Source: three-view drawing plus pictorial views. Frame: mm from the lowest corner of the part. A direction names the side the tool comes from. Give positions to 0.01 mm unless a question says otherwise; leave off trailing zeros. Loops run counter-clockwise (first coordinate to the right, second up) from the corner with the lowest first, then second, coordinate; pieces in that order, holes last.
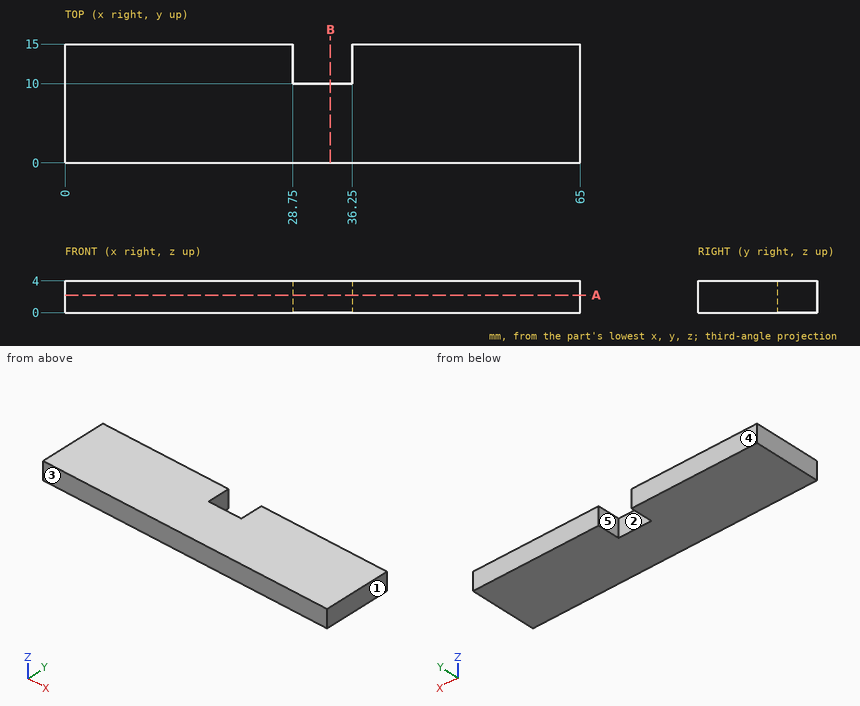
(1) Mould query, pull axis X, two halves, no side actions, for the marked faces 1, 2 and 3. Classes: +X half, -X half, draft (parallel to the pull), parting line (faces both ways), or undercut.
Values follow:
face 1: +X half
face 2: undercut
face 3: draft
(2) Ray query, probe 1 along X at (y, z) = (14, 1.95). Return the intervals inside material, ascending.
Values follow:
probe 1: x = 0 to 28.75, 36.25 to 65
(3) Reachability of the marked faces 4 and 5 from +Z, -Z, +X, -X, +Y, -Y: full face, straight path, thin tool, end or side. Return the list, or none.
Values follow:
face 4: +Z, -Z, +X, -X, +Y
face 5: +Z, -Z, +Y
(4) Cut plane A-A (z = 2.2). Return the cut outline in (x, y), and give its area (4 significant figures).
Values follow:
outline: (0, 0) - (65, 0) - (65, 15) - (36.25, 15) - (36.25, 10) - (28.75, 10) - (28.75, 15) - (0, 15) - close
area: 937.5 mm2
(5) Cut plane B-B (x = 33.5). Return the cut outline in (y, z).
Values follow:
outline: (0, 0) - (10, 0) - (10, 4) - (0, 4) - close
